Work out the finished part from the listing and answer in its coordinate system (mm). A direction names the side the tool comes from. Give positions to 0.01 mm unless a question says otherwise; leave off trailing zeros. Write each loop counter-clockwise with the first axis right and the second up, starting at its lowest first coordinate (ties: lowest second). Pieces come first, ordered by that corner, then holes.
1) Straight lines are drawn through the part: probe 1 along Z at (x, y) = (1, 2.5); probe 2 along Y at (x, z) = (27, -6.5) (3 decimals); probe 3 along Y at (x, z) = (9.5, -7) (3 decimals). For each, find the intervals that lie inside material, in ascending order.
2) Find section B-B (y = 3). Determine the outline of the cut face in (x, z) (3 decimals).
3) Determine the mould class of faces 4 (the face through (5.343, -6.306, -0.478)), 5 (the face through (6, 3, 3.013)), 6 (the face through (2.3, 6.35, 3.3)) for opening direction Z: pulls with the +Z half, pulls with the -Z half, needs draft (parallel to the pull), parting line crosses it, or undercut.
4) Find section D-D (y = -5.5). Determine the outline of the cut face in (x, z) (3 decimals).
5) Find section C-C (z = -3.75). Determine the outline of the cut face in (x, y) (3 decimals), plus the area to 3 significant figures.
6) Given pin 1 Ø2 at (y, z) = (3.5, 3.5) entering from +X; pin 2 Ø3 at (x, z) = (10, 1.5) entering from -Y (3 decimals); pin 3 Ø1 at (y, z) = (-8, -2.5) entering from +X, each flat-ended and moving along its own axis, determine where each tip first touches the part or whether it passes through.
7) Find section A-A (x = -2). Determine the outline of the cut face in (y, z) (3 decimals), plus the area to 3 significant figures.
8) A tool of negligible diameter and unlimited length cuts with its end or side. For faces 1 (the face through (-9.431, 1.521, 4.013)), 2 (the face through (16.919, 3, -7)), 3 (the face through (6, 3, -5.877)), from which of +Z, -Z, +X, -X, +Y, -Y can it reach the whole face along a straight path? Write none if from no direction.
```python
from build123d import *

# Parameters (mm, degrees)
F0_W     = 50.8
F0_H     = 12.7
F1_DEPTH = 3.175
F2_R     = 3.175
F3_DEPTH = 6.35
F5_DEPTH = 6.35
F6_R     = 6.34999
F7_R     = 3.175


# Not quite as in the source:
# - a fillet or chamfer is up to 0.001 mm smaller than in the source, because OpenCascade refuses the exact size


with BuildPart() as f1:
    # F0 (on Front) → F1 (new body)
    with BuildSketch(Plane.XZ):
        with Locations((15.0143924374, -1.4320164919)):
            Rectangle(F0_W, F0_H)
    extrude(amount=F1_DEPTH)

    # F2 (on face) → F3 (join)
    with BuildSketch(Plane.XZ.offset(3.175)):
        with Locations((2.3143924374, -1.4320164919)):
            Circle(F2_R)
    extrude(amount=F3_DEPTH)

    # F4 (on face) → F5 (join)
    with BuildSketch(Plane(origin=(0, 0, 0), x_dir=(-1, 0, 0), z_dir=(0, 1, 0))):
        Polygon((8.4806075626, 3.0129835081), (8.4806075626, -5.8770164919), (-16.9193924374, -5.8770164919), (-16.9193924374, -7.7820164919), (10.3856075626, -7.7820164919), (10.3856075626, 4.9179835081), (-16.9193924374, 4.9179835081), (-16.9193924374, 3.0129835081), align=None)
    extrude(amount=F5_DEPTH)

    # F6 (radius 6.35 in the source; OpenCascade refuses exactly that, so slightly less here)
    f6_edges = [f1.edges().sort_by_distance(p)[0] for p in [
        (40.414392, -1.5875, 4.917984),
        (40.414392, -1.5875, -7.782016),
    ]]
    fillet(f6_edges, radius=F6_R)

    # F7
    f7_edges = [f1.edges().sort_by_distance(p)[0] for p in [
        (-8.480608, 3.175, 3.012984),
        (-8.480608, 3.175, -5.877016),
        (-10.385608, 1.5875, 4.917984),
        (-10.385608, 1.5875, -7.782016),
    ]]
    fillet(f7_edges, radius=F7_R)


solid = f1.part
```
Results:
1. probe 1: z = -7.78 to -5.88, 3.01 to 4.92
1. probe 2: y = -3.175 to 0
1. probe 3: y = -3.175 to 6.35
2. outline: (-10.386, -4.607) arc R3.175 ccw to (-7.211, -7.782) - (16.919, -7.782) - (16.919, -5.877) - (-5.306, -5.877) arc R3.175 cw to (-8.481, -2.702) - (-8.481, -0.162) arc R3.175 cw to (-5.306, 3.013) - (16.919, 3.013) - (16.919, 4.918) - (-7.211, 4.918) arc R3.175 ccw to (-10.386, 1.743) - close
3. face 4: parting line crosses it
3. face 5: undercut
3. face 6: needs draft
4. outline: circle Ø6.35 at (2.314, -1.432)
5. outline: (-10.386, -3.175) - (0.145, -3.175) - (0.145, -9.525) - (4.484, -9.525) - (4.484, -3.175) - (39.976, -3.175) - (39.976, 0) - (-8.303, 0) - (-8.303, 6.35) - (-10.386, 6.35) - close
5. area: 201 mm2
6. pin 1: stops at x = 16.92
6. pin 2: stops at y = -3.175
6. pin 3: stops at x = 5.44
7. outline: (-3.175, -7.782) - (6.35, -7.782) - (6.35, -5.877) - (0, -5.877) - (0, 3.013) - (6.35, 3.013) - (6.35, 4.918) - (-3.175, 4.918) - close
7. area: 64.5 mm2
8. face 1: +Z, -X, +Y, -Y
8. face 2: +Z, -Z, +X, +Y
8. face 3: +X, +Y
